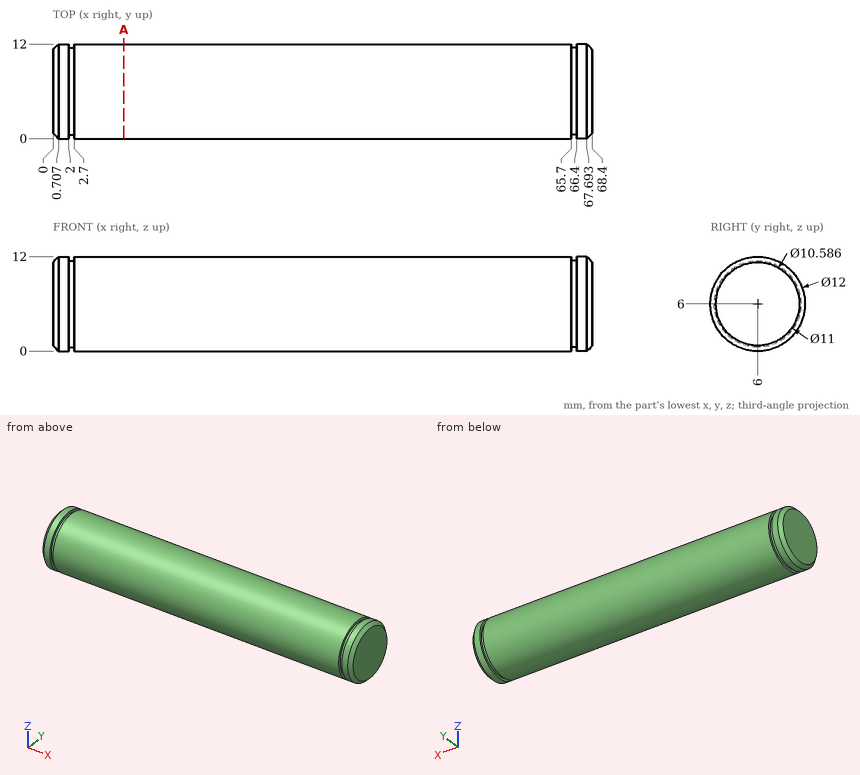
Geometry check sheet. Reference: drawing and pictorial views, mm from the part's lowest x, y, z. Round coordinates to 2 decimals unless told otherwise and drop trailing zeros. Loops run counter-clockwise (first coordinate to the right, second up) from the corner with the lowest first, then second, coordinate; pieces in that order, holes last. Notation, with made-up numbers: (80, 26) - (100, 26) arc R29 cw to (100, 55) - close; hole circle Ø4 at (83.25, 53.5). An arc over 180 degrees is marked (long way). Write item = value, one per line. Start each with the question number.
Q1. Depth check by flat-ended pin: P1, Ø1.5, axis at x = 9, z = 8.5, coming from the -Y side; P2, Ø1, axis at x = 58.5, z = 5, coming from the -Y side; P3, Ø1.5, axis at x = 35, z = 2.5, coming from the -Y side. Enter the tip coordinate at first touch or a pass-through.
Q2. Section check A-A (x = 9). Record the boundary of the cut face in (y, z), plus the area to 3 significant figures.
Q3. Thickness scan on L1, parallel to Y at x = 13.5, z = 3.5 (1 decimal); L2, parallel to Z at x = 11, y = 10.5; L3, parallel to Y at x = 31, z = 1. Record the ranges inside material, lowest first.
Derived:
q1.P1 = 0.26
q1.P2 = 0.02
q1.P3 = 0.67
q2.outline = circle Ø12 at (6, 6)
q2.area = 113 mm^2
q3.L1 = 0.5 to 11.5
q3.L2 = 2.03 to 9.97
q3.L3 = 2.68 to 9.32
